```python
from build123d import *

# Parameters (mm, degrees)
ESQUISSE1_W             = 600
ESQUISSE1_H             = 16.28
BOSS_EXTRU_1_DEPTH      = 100
CHANFREIN1_SIZE         = 2
ENL_V_START             = -53
ENL_V_MAT_EXTRU_1_DEPTH = 48
ENL_V_START_2           = 53
ENL_V_MAT_EXTRU_2_DEPTH = 48
ENL_V_START_3           = 100
ENL_V_MAT_EXTRU_4_DEPTH = 30


with BuildPart() as part:
    # Esquisse1 → Boss.-Extru.1 (new body, symmetric)
    with BuildSketch(Plane.XY):
        with Locations((300, 8.14)):
            Rectangle(ESQUISSE1_W, ESQUISSE1_H)
    extrude(amount=BOSS_EXTRU_1_DEPTH, both=True)

    # Chanfrein1
    chanfrein1_edges = [part.edges().sort_by_distance(p)[0] for p in [
        (600, 16.28, 0),
        (600, 0, 0),
        (0, 0, 0),
        (0, 16.28, 0),
    ]]
    chamfer(chanfrein1_edges, length=CHANFREIN1_SIZE)

    # Esquisse1_4 → Enl_v. mat.-Extru.1 (cut, through all)
    with BuildSketch(Plane.XY.offset(ENL_V_START)):
        Polygon((105, 16.28), (125, 16.28), (125, 11.28), (132.5, 11.28), (132.5, 6.28), (97.5, 6.28), (97.5, 11.28), (105, 11.28), align=None)
        Polygon((425, 16.28), (445, 16.28), (445, 11.28), (452.5, 11.28), (452.5, 6.28), (417.5, 6.28), (417.5, 11.28), (425, 11.28), align=None)
    extrude(amount=-ENL_V_MAT_EXTRU_1_DEPTH, mode=Mode.SUBTRACT)

    # Esquisse1_5 → Enl_v. mat.-Extru.2 (cut, through all)
    with BuildSketch(Plane.XY.offset(ENL_V_START_2)):
        Polygon((105, 16.28), (125, 16.28), (125, 11.28), (132.5, 11.28), (132.5, 6.28), (97.5, 6.28), (97.5, 11.28), (105, 11.28), align=None)
        Polygon((425, 16.28), (445, 16.28), (445, 11.28), (452.5, 11.28), (452.5, 6.28), (417.5, 6.28), (417.5, 11.28), (425, 11.28), align=None)
    extrude(amount=ENL_V_MAT_EXTRU_2_DEPTH, mode=Mode.SUBTRACT)

    # Esquisse1_9 → Enl_v. mat.-Extru.4 (cut)
    with BuildSketch(Plane.XY.offset(ENL_V_START_3)):
        Polygon((585, 11.28), (585, 16.28), (565, 16.28), (565, 11.28), (557.5, 11.28), (557.5, 6.28), (592.5, 6.28), (592.5, 11.28), align=None)
    extrude(amount=-ENL_V_MAT_EXTRU_4_DEPTH, mode=Mode.SUBTRACT)


solid = part.part
```
Can you work these out from the model? Positions are in its coordinate system, mm. A direction names the side the tool comes from. Coordinates: 2 decimals unless noted, no trailing zeros. Order: outer loops, then holes, each group sorted by start corner. A loop starts at its lowest first (then second) coordinate and runs counter-clockwise, first axis right, second up.
1. I need wall thicknesses on line 1 (X direction, y = 8.75, z = 55); line 2 (X direction, y = 13.25, z = 88); line 3 (X direction, y = 11.75, z = -77.5). Which ranges of each line are inside material? Lowest first, please.
2. I'm going to push a flat-ended pin straight in: pin 1 (5 mm diameter, centred on x = 108.5, z = -67.5, fed in from +Y). Where does the tip first touch, or does it pass through?
3. If we section it at A-A (x = 437): Please give me the cut outline in (y, z), then the cut area to 3 significant figures.
4. For faces 4 (the face through (296, 16.28, 1)), 5 (the face through (115, 6.28, -76)), 6 (the face through (115, 6.28, 76)), which set-ups out of +Z, -Z, +X, -X, +Y, -Y let a thin tool reach every point of the face, with its end or its side?
5. Thinking about a two-plate mould opening in Y: for faces 1 (the face through (435, 6.28, 76)), 2 (the face through (600, 8, 1)), 3 (the face through (296, 0, 1)), which applies, +Y half, -Y half, draft (parallel to the pull), parting line (faces both ways), or undercut?
Entries:
1. line 1: x = 0 to 97.5, 132.5 to 417.5, 452.5 to 600
1. line 2: x = 0 to 105, 125 to 425, 445 to 565, 585 to 600
1. line 3: x = 0 to 105, 125 to 425, 445 to 600
2. pin 1: stops at y = 6.28
3. outline: (0, -100) - (6.28, -100) - (6.28, -53) - (16.28, -53) - (16.28, 53) - (6.28, 53) - (6.28, 100) - (0, 100) - close
3. area: 2,320 mm2
4. face 4: +Z, -Z, +X, -X, +Y
4. face 5: -Z
4. face 6: +Z
5. face 1: undercut
5. face 2: draft
5. face 3: -Y half
